Autodesk Inventor part; units mm, degrees
ref_plane "YZ Plane" through (0, 0, 0) normal (1, 0, 0) x (0, 1, 0)
ref_plane "XZ Plane" through (0, 0, 0) normal (0, 1, 0) x (-1, 0, 0)
ref_plane "XY Plane" through (0, 0, 0) normal (0, 0, 1) x (1, 0, 0)
sketch "Sketch1" plane through (0, 0, 0) normal (0, 0, 1) x (1, 0, 0)
  line L0 (-25.4, 6.35) -> (-25.4, 0)
  line L1 (-25.4, 0) -> (-4.7625, 0)
  line L2 (-4.7625, 0) -> (-4.7625, 6.35)
  line L3 (-4.7625, 6.35) -> (-25.4, 6.35)
  dimension "d0" = 6.35
  dimension "d1" = 20.6375
extrude "Extrusion1" add sketch "Sketch1" along normal blind 3.175
hole "Hole1" at (-9.525, 3.175, 3.175) direction (0, 0, -1) diameter 4.318 end through all
chamfer "Chamfer3" distance 0.7937 angle 45 1 edges at (-4.7625, 0, 1.5875)
chamfer "Chamfer4" distance 0.7937 angle 45 1 edges at (-4.7625, 6.35, 1.5875)
chamfer "Chamfer5" distance 0.7937 distance2 3.175 1 edges at (-25.4, 0, 1.5875) measured on face at (-25.4, 4.2333, 1.0583)
chamfer "Chamfer6" distance 3.175 distance2 0.7937 1 edges at (-25.4, 6.35, 1.5875) measured on face at (-12.1708, 6.35, 1.0583)
chamfer "Chamfer7" distance 6.096 angle 15 1 edges at (-25.4, 3.175, 3.175) measured on face at (-18.7061, 3.2617, 3.175)
fillet "Fillet1" radius 0.635 2 edges at (-25.4, 0.7937, 0.7708) (-25.4, 5.5562, 0.7708)
properties part number "J005776" material "STAINLESS STEEL, 303"
Geometry check sheet. Reference: the model listing, model coordinates, mm. Round coordinates to 2 decimals unless told otherwise and drop trailing zeros. Loops run counter-clockwise (first coordinate to the right, second up) from the corner with the lowest first, then second, coordinate; pieces in that order, holes last. Notation, with made-up numbers: (70.5, 53) - (127.5, 53) arc R8 ccw to (127.5, 62) - close; hole circle Ø2 at (89.25, 26). An arc over 180 degrees is marked (long way). Write each question's results on one line, items separated by ' | '. Start each with the question number.
Q1. Release check for a two-part mould opening along X. For faces 1 (the flat face through (-23.59, 6.01, 0.95)), 2 (the flat face through (-12, 3, 3.175)), 3 (the cylindrical face through (-11.666, 3.456, 1.565)) record: +X half, -X half, draft (parallel to the pull), parting line (faces both ways), or undercut.
Q2. Thickness scan on line 1 (X direction, y = 4.5, z = 0.95); line 2 (X direction, y = 4, z = 0.6); line 3 (Y direction, x = -11.5, z = 2.75). Record the ranges inside material, lowest first. Write a range as [from, to].
Q3. Cross-section at A-A on x = -8.75. Enter the section's corners in (y, z) (3 decimals), and give its area (3 significant figures).
Q4. Cross-section at B-B on y = 1.5. Enter the section's corners in (x, z) (1 decimal).
Answers below:
1) face 1: -X half | face 2: draft | face 3: undercut
2) line 1: x = [-25.4, -11.23], [-7.82, -4.76] | line 2: x = [-25.4, -11.52], [-7.53, -4.76] | line 3: y = [0, 2.3], [4.05, 6.35]
3) outline: (0, 0) - (1.16, 0) - (1.16, 3.175) - (0, 3.175) - close; (5.19, 0) - (6.35, 0) - (6.35, 3.175) - (5.19, 3.175) - close | area: 7.37 mm²
4) outline: (-25.4, 0) - (-10.9, 0) - (-10.9, 3.2) - (-19.3, 3.2) - (-25.4, 1.5) - close; (-8.2, 0) - (-4.8, 0) - (-4.8, 3.2) - (-8.2, 3.2) - close
